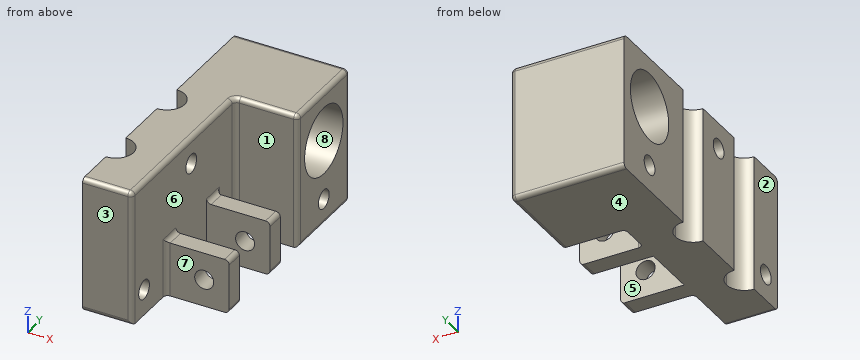
```python
from build123d import *

# Parameters (mm, degrees)
F0_W     = 14
F0_H     = 20
F1_DEPTH = 30
F0_H_2   = 4
F2_DEPTH = 12
F3_R     = 7.5
F3_R_2   = 2.1
F4_DEPTH = 25.001
F5_R     = 2.1
F6_DEPTH = 25
F7_R     = 1


with BuildPart() as f1:
    # F0 (on Top) → F1 (new body)
    with BuildSketch(Plane.XY):
        with BuildLine():
            Line((-28.710388, 64.3535), (-39.710388, 64.3535))
            Line((-39.710388, 64.3535), (-39.710388, 41.2535))
            ThreePointArc((-39.710388, 41.2535), (-36.952671, 40.111216), (-35.810388, 37.3535))
            ThreePointArc((-35.810388, 37.3535), (-36.952671, 34.595783), (-39.710388, 33.4535))
            Line((-39.710388, 33.4535), (-39.710388, 21.2535))
            ThreePointArc((-39.710388, 21.2535), (-36.952671, 20.111216), (-35.810388, 17.3535))
            ThreePointArc((-35.810388, 17.3535), (-36.952671, 14.595783), (-39.710388, 13.4535))
            Line((-39.710388, 13.4535), (-39.710388, 4.3535))
            Line((-39.710388, 4.3535), (-28.710388, 4.3535))
            Line((-28.710388, 4.3535), (-28.710388, 17.3535))
            Line((-28.710388, 17.3535), (-28.710388, 21.3535))
            Line((-28.710388, 21.3535), (-28.710388, 33.3535))
            Line((-28.710388, 33.3535), (-28.710388, 37.3535))
            Line((-28.710388, 37.3535), (-28.710388, 44.3535))
            Line((-28.710388, 44.3535), (-28.710388, 64.3535))
        make_face()
        with Locations((-21.710388, 54.3535)):
            Rectangle(F0_W, F0_H)
    extrude(amount=F1_DEPTH)

    # F0 (on Top) → F2 (join)
    with BuildSketch(Plane.XY):
        with Locations((-21.710388, 35.3535)):
            Rectangle(F0_W, F0_H_2)
        with Locations((-21.710388, 19.3535)):
            Rectangle(F0_W, F0_H_2)
    extrude(amount=F2_DEPTH)

    # F3 (on face) → F4 (cut, through all)
    with BuildSketch(Plane.YZ.offset(-14.710388)):
        with Locations((54.3535, 19)):
            Circle(F3_R)
        with Locations((54.3535, 5.75)):
            Circle(F3_R_2)
        with Locations((27.3535, 24.25)):
            Circle(F3_R_2)
        with Locations((8.9035, 5.75)):
            Circle(F3_R_2)
    extrude(amount=-F4_DEPTH, mode=Mode.SUBTRACT)

    # F5 (on face) → F6 (cut)
    with BuildSketch(Plane(origin=(0, 37.3535, 0), x_dir=(-1, 0, 0), z_dir=(0, 1, 0))):
        with Locations((20.210388, 6)):
            Circle(F5_R)
    extrude(amount=-F6_DEPTH, mode=Mode.SUBTRACT)

    # F7
    f7_edges = [f1.edges().sort_by_distance(p)[0] for p in [
        (-14.710388, 35.3535, 12),
        (-14.710388, 19.3535, 12),
        (-14.710388, 19.3535, 0),
        (-14.710388, 54.3535, 0),
        (-14.710388, 44.3535, 15),
        (-14.710388, 54.3535, 30),
        (-14.710388, 64.3535, 15),
        (-27.210388, 64.3535, 0),
        (-27.210388, 64.3535, 30),
        (-34.210388, 4.3535, 0),
        (-28.710388, 4.3535, 15),
        (-28.710388, 24.3535, 30),
        (-21.710388, 44.3535, 30),
        (-28.710388, 19.3535, 12),
        (-28.710388, 35.3535, 12),
        (-28.710388, 37.3535, 6),
        (-28.710388, 17.3535, 6),
        (-34.210388, 4.3535, 30),
        (-28.710388, 44.3535, 15),
        (-14.710388, 35.3535, 0),
    ]]
    fillet(f7_edges, radius=F7_R)


solid = f1.part
```
Design review of the part built by this model. Coordinates are the model's own, in mm. Face numbers are marked on the shaded views. A direction names the side the tool comes from. Coordinates: 2 decimals unless noted, no trailing zeros. Order: outer loops, then holes, each group sorted by start corner. A loop starts at its lowest first (then second) coordinate and runs counter-clockwise, first axis right, second up. Notation, with made-up numbers: M 69,78.25 L 92,78.25 A10 ccw 92,96.25 Z; hole C 0,74 d5. An arc over 180 degrees is marked long. Answer as a JSON object with one key per item and string values. Group by question number.
1) Mouldability with a two-part tool opening along Y and no side actions: class the marked faces 1, 2 and 3 as pulls with the +Y half, pulls with the -Y half, needs draft (parallel to the pull), parting line crosses it, or undercut.
2) For pin 1 (5.5 mm diameter, centred on y = 27.35, z = 24.25, fed in from +X); pin 2 (6.5 mm diameter, centred on x = -22.5, z = 8, fed in from -Y); pin 3 (3 mm diameter, centred on x = -22.5, y = 19, fed in from +Z); pin 4 (3.5 mm diameter, centred on y = 54.35, z = 5.75, fed in from -X), all flat-tipped, find the tip position at first contact; note any pin that passes through.
3) Add section C-C, the plane z = 19. Write out the cut boundary in (x, y).
4) Add section A-A, the plane x = -16.5. Write out the cut boundary in (y, z), then the cut area to 3 significant figures.
5) Wall thickness on L1, parallel to Y at x = -26, z = 3; L2, parallel to X at y = 10.5, z = 1.75; L3, parallel to Y at x = -21.5, z = 24.5: over which ranges is each line inside the solid? List them lowest first.
6) Add section D-D, the plane x = -35. Write out the cut boundary in (y, z).
7) Add section B-B, the plane x = -21. Write out the cut boundary in (y, z).
8) Tool access review of the marked faces 4, 5, 6, 7 and 8: name each direction out of +Z, -Z, +X, -X, +Y, -Y from which nothing blocks a thin tool from reaching the whole face with its end or side.
Computed values:
{
 "1": {"face 1": "undercut", "face 2": "needs draft", "face 3": "pulls with the -Y half"},
 "2": {"pin 1": "stops at x = -28.71", "pin 2": "stops at y = 17.35", "pin 3": "stops at z = 12", "pin 4": "passes through"},
 "3": {"outline": "M -39.71,4.35 L -29.71,4.35 A1 ccw -28.71,5.35 L -28.71,43.35 A1 cw -27.71,44.35 L -15.71,44.35 A1 ccw -14.71,45.35 L -14.71,46.85 L -39.71,46.85 L -39.71,41.25 A3.9 cw -35.81,37.35 A3.9 cw -39.71,33.45 L -39.71,21.25 A3.9 cw -35.81,17.35 A3.9 cw -39.71,13.45 Z; M -39.71,61.85 L -14.71,61.85 L -14.71,63.35 A1 ccw -15.71,64.35 L -39.71,64.35 Z"},
 "4": {"outline": "M 17.35,0 L 21.35,0 L 21.35,12 L 17.35,12 Z; M 33.35,0 L 37.35,0 L 37.35,12 L 33.35,12 Z; M 44.35,0 L 63.35,0 A1 ccw 64.35,1 L 64.35,29 A1 ccw 63.35,30 L 45.35,30 A1 ccw 44.35,29 Z; hole C 54.35,19 d15; hole C 54.35,5.75 d4.2", "area": "505 mm^2"},
 "5": {"L1": "y = 17.35 to 21.35, 33.35 to 37.35, 44.35 to 64.35", "L2": "x = -39.71 to -28.71", "L3": "y = 44.35 to 49.25, 59.45 to 64.35"},
 "6": {"outline": "M 4.35,1 A1 ccw 5.35,0 L 63.35,0 A1 ccw 64.35,1 L 64.35,29 A1 ccw 63.35,30 L 5.35,30 A1 ccw 4.35,29 Z; hole C 8.9,5.75 d4.2; hole C 27.35,24.25 d4.2; hole C 54.35,19 d15; hole C 54.35,5.75 d4.2"},
 "7": {"outline": "M 17.35,0 L 21.35,0 L 21.35,4.05 L 17.35,4.05 Z; M 17.35,7.95 L 21.35,7.95 L 21.35,12 L 17.35,12 Z; M 33.35,0 L 37.35,0 L 37.35,4.05 L 33.35,4.05 Z; M 33.35,7.95 L 37.35,7.95 L 37.35,12 L 33.35,12 Z; M 44.35,0 L 63.35,0 A1 ccw 64.35,1 L 64.35,29 A1 ccw 63.35,30 L 45.35,30 A1 ccw 44.35,29 Z; hole C 54.35,19 d15; hole C 54.35,5.75 d4.2"},
 "8": {"face 4": "-Z, +X, -X, +Y, -Y", "face 5": "+Z, -Z, +X", "face 6": "+Z, +X", "face 7": "+Z, -Z, +X, -Y", "face 8": "+X, -X"}
}
